Read the model definition and answer for the solid it produces. Units are mm, in the model's axes. Coordinates: 2 decimals unless noted, no trailing zeros. Order: outer loops, then holes, each group sorted by start corner. A loop starts at its lowest first (then second) coordinate and runs counter-clockwise, first axis right, second up. Notation, with made-up numbers: M -7.5,-1 L 36.5,-1 A27 ccw 36.5,18 Z; hole C 55,29.5 d9. An arc over 180 degrees is marked long. Use a Markdown table: item, result. Add a question column.
1) Each of these flat-tipped pins is pushed along its axis until it touches: pin 1 Ø3 at (x, z) = (22, 4) entering from -Y; pin 2 Ø3 at (y, z) = (-8.5, 4.5) entering from -X; pin 3 Ø1.5 at (x, z) = (25, 5) entering from +Y. Where does it stop, or does it pass through?
2) Find section B-B on x = 80. Write down the section's boundary in (y, z), plus the area to 3 significant figures.
3) Find the intervals of material crossed by probe 1 along Y at (x, z) = (0, 3.85); probe 2 along X at (y, z) = (-10, 5.6); probe 3 along Y at (x, z) = (-80, 3.8), in increasing order. Write a range as [from, to].
4) Find section A-A on y = 0. Write down the section's boundary in (x, z).
5) Find section C-C on z = 1.95. Write down the section's boundary in (x, y), plus the area to 3 significant figures.
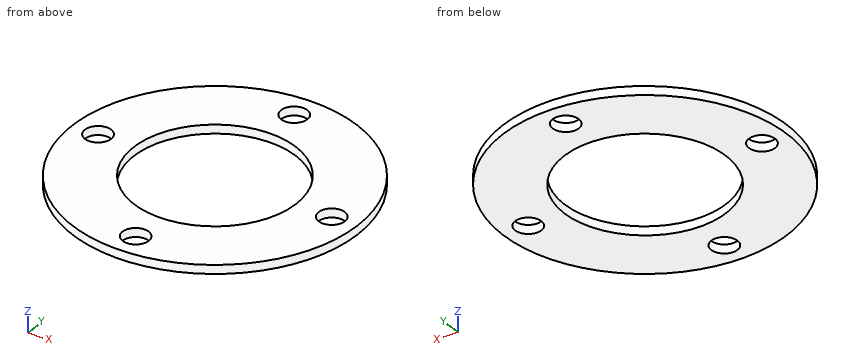
Autodesk Inventor part; units mm, degrees
ref_plane "YZ Plane" through (0, 0, 0) normal (1, 0, 0) x (0, 1, 0)
ref_plane "XZ Plane" through (0, 0, 0) normal (0, 1, 0) x (-1, 0, 0)
ref_plane "XY Plane" through (0, 0, 0) normal (0, 0, 1) x (1, 0, 0)
sketch "Sketch2" plane through (0, 0, 0) normal (0, 0, 1) x (1, 0, 0)
  circle A0 centre (0, 0) radius 55.5
  circle A1 centre (0, 0) radius 97.5
  circle A2 centre (0, 0) radius 80 construction
  circle A3 centre (0, 80) radius 9
  circle A4 centre (-80, 0) radius 9
  circle A5 centre (0, -80) radius 9
  circle A6 centre (80, 0) radius 9
  dimension "d29" = 160
  dimension "d25" = 111
  dimension "d27" = 195
  dimension "d30" = 18
  dimension "d33" = 360
extrude "Plate2" add sketch "Sketch2" along normal blind 6
equation "\"d14\" = Thickness"
equation "\"BendReliefWidth\" = Thickness"
equation "\"BendReliefDepth\" = 0.5 * Thickness"
equation "\"CornerReliefSize\" = 4 * Thickness"
equation "\"MinimumRemnant\" = 2 * Thickness"
equation "\"TransitionRadius\" = BendRadius"
equation "\"JacobiRadiusSize\" = BendRadius"
equation "\"GapSize\" = Thickness"
properties part number "PRS 1200-31 FDS flange DN90" material "Steel"
Check result:
| question | item | result |
|---|---|---|
| 1 | pin 1 | stops at y = -95.32 |
| 1 | pin 2 | stops at x = -97.25 |
| 1 | pin 3 | stops at y = 94.44 |
| 2 | outline | M -55.73,0 L -9,0 L -9,6 L -55.73,6 Z; M 9,0 L 55.73,0 L 55.73,6 L 9,6 Z |
| 2 | area | 561 mm2 |
| 3 | probe 1 | y = [-97.5, -89], [-71, -55.5], [55.5, 71], [89, 97.5] |
| 3 | probe 2 | x = [-96.99, -54.59], [54.59, 96.99] |
| 3 | probe 3 | y = [-55.73, -9], [9, 55.73] |
| 4 | outline | M -97.5,0 L -89,0 L -89,6 L -97.5,6 Z; M -71,0 L -55.5,0 L -55.5,6 L -71,6 Z; M 55.5,0 L 71,0 L 71,6 L 55.5,6 Z; M 89,0 L 97.5,0 L 97.5,6 L 89,6 Z |
| 5 | outline | C 0,0 d195; hole C -80,0 d18; hole C 0,0 d111; hole C 0,-80 d18; hole C 0,80 d18; hole C 80,0 d18 |
| 5 | area | 19,200 mm2 |
